Print and shaded views of the part. All mm, measured from the part's lowest x, y and z. A direction names the side the tool comes from. Round coordinates to 2 decimals unless told otherwise and drop trailing zeros. Loops run counter-clockwise (first coordinate to the right, second up) from the corner with the lowest first, then second, coordinate; pieces in that order, holes last. Notation, with made-up numbers: (-16.75, -26.75) - (17.25, -26.75) arc R26 cw to (17.25, 12.25) - close; hole circle Ø10 at (76, -15). An arc over 180 degrees is marked (long way). Use one line per item in the form item = value.
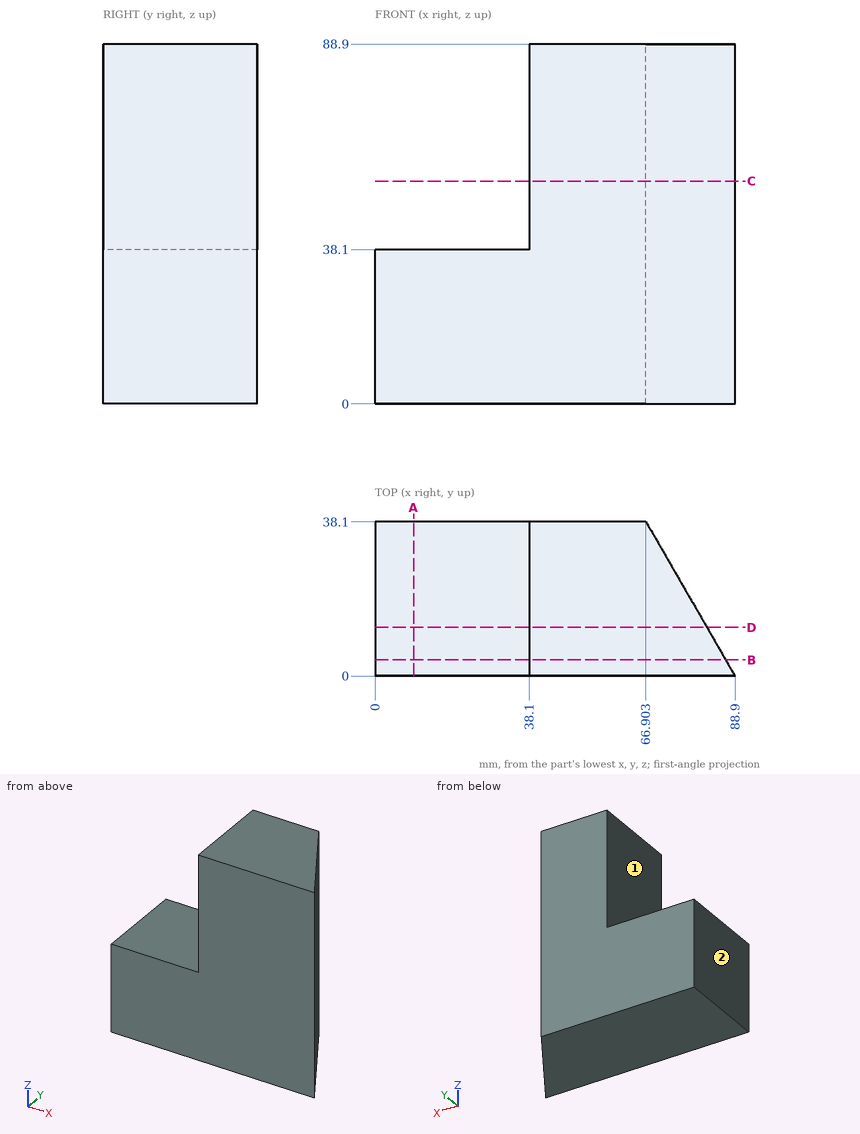
1. Cut at D-D, the plane y = 12. Give the cut face in (x, z), plus the area to 3 significant figures.
Geometry check:
outline = (0, 0) - (81.97, 0) - (81.97, 88.9) - (38.1, 88.9) - (38.1, 38.1) - (0, 38.1) - close
area = 5,350 mm^2
2. Wall check: probe 1 along Z at (x, y) = (22.5, 10); probe 2 along X at (y, z) = (11, 44); probe 3 along X at (y, z) = (31, 32.5). Give the ranges that are in metal, low to high.
Geometry check:
probe_1 = 0 to 38.1
probe_2 = 38.1 to 82.55
probe_3 = 0 to 71
3. Cut at C-C, the plane z = 55. Give the cut face in (x, y).
Geometry check:
outline = (38.1, 0) - (88.9, 0) - (66.9, 38.1) - (38.1, 38.1) - close
4. Cut at A-A, the plane x = 9.5. Give the cut face in (y, z), plus the area to 3 significant figures.
Geometry check:
outline = (0, 0) - (38.1, 0) - (38.1, 38.1) - (0, 38.1) - close
area = 1,450 mm^2
5. Tool access for the marked faces 1 and 2: list every direction of +Z, -Z, +X, -X, +Y, -Y with a clear straight run to the whole face (end or side of a thin tool).
Geometry check:
face_1 = +Z, -X, +Y, -Y
face_2 = +Z, -Z, -X, +Y, -Y
6. Flat gauge pins, fed straight in: pin 1 (3 mm diameter, centred on x = 32.5, y = 7, fed in from +Z); pin 2 (2 mm diameter, centred on x = 70, z = 17, fed in from +Y); pin 3 (1 mm diameter, centred on x = 26.5, y = 22, fed in from -Z); pin 4 (3 mm diameter, centred on y = 24, z = 58, fed in from +X). Where does each tip first touch, or does it go through?
Geometry check:
pin_1 = 38.1
pin_2 = 34.47
pin_3 = 0
pin_4 = 75.91
7. Cut at B-B, the plane y = 4. Give the cut face in (x, z).
Geometry check:
outline = (0, 0) - (86.59, 0) - (86.59, 88.9) - (38.1, 88.9) - (38.1, 38.1) - (0, 38.1) - close
